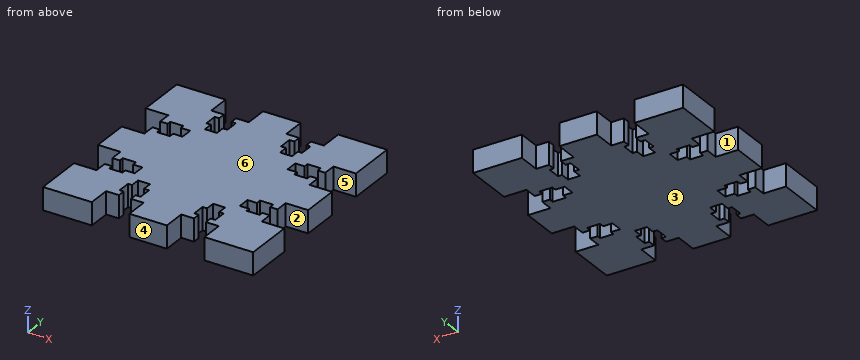
from build123d import *

# Parameters (mm, degrees)
SKETCH1_W           = 56
SKETCH1_H           = 56
BOSS_EXTRUDE1_DEPTH = 6
SKETCH2_W           = 10
SKETCH2_H           = 6
SKETCH2_W_2         = 6
SKETCH2_H_2         = 10
CUT_EXTRUDE1_DEPTH  = 54.425204723
SKETCH4_W           = 3.2
SKETCH4_H           = 6
CUT_EXTRUDE2_DEPTH  = 8
SKETCH10_W          = 6
SKETCH10_H          = 3.2
CUT_EXTRUDE7_DEPTH  = 8
SKETCH11_W          = 3.2
SKETCH11_H          = 6
CUT_EXTRUDE8_DEPTH  = 8
SKETCH12_W          = 6
SKETCH12_H          = 3.2
CUT_EXTRUDE9_DEPTH  = 8
SKETCH13_W          = 3.5
SKETCH13_H          = 5.6
SKETCH13_W_2        = 5.6
SKETCH13_H_2        = 3.5
CUT_EXTRUDE10_DEPTH = 54.425204723


with BuildPart() as part:
    # Sketch1 → Boss-Extrude1 (new body)
    with BuildSketch(Plane.XY):
        with Locations((6.733082315, -12.148044693)):
            Rectangle(SKETCH1_W, SKETCH1_H)
    extrude(amount=BOSS_EXTRUDE1_DEPTH)

    # Sketch2 → Cut-Extrude1 (cut, through all)
    with BuildSketch(Plane.XY.offset(6)):
        with Locations((-3.266917685, 12.851955307)):
            Rectangle(SKETCH2_W, SKETCH2_H)
        with Locations((16.733082315, 12.851955307)):
            Rectangle(SKETCH2_W, SKETCH2_H)
        with Locations((31.733082315, -2.148044693)):
            Rectangle(SKETCH2_W_2, SKETCH2_H_2)
        with Locations((31.733082315, -22.148044693)):
            Rectangle(SKETCH2_W_2, SKETCH2_H_2)
        with Locations((16.733082315, -37.148044693)):
            Rectangle(SKETCH2_W, SKETCH2_H)
        with Locations((-3.266917685, -37.148044693)):
            Rectangle(SKETCH2_W, SKETCH2_H)
        with Locations((-18.266917685, -22.148044693)):
            Rectangle(SKETCH2_W_2, SKETCH2_H_2)
        with Locations((-18.266917685, -2.148044693)):
            Rectangle(SKETCH2_W_2, SKETCH2_H_2)
    extrude(amount=-CUT_EXTRUDE1_DEPTH, mode=Mode.SUBTRACT)

    # Sketch4 → Cut-Extrude2 (cut)
    with BuildSketch(Plane(origin=(0, 9.851955307, 0), x_dir=(1, 0, 0), z_dir=(0, 1, 0))):
        with Locations((16.733082315, -3)):
            Rectangle(SKETCH4_W, SKETCH4_H)
        with Locations((-3.266917685, -3)):
            Rectangle(SKETCH4_W, SKETCH4_H)
    extrude(amount=-CUT_EXTRUDE2_DEPTH, mode=Mode.SUBTRACT)

    # Sketch10 → Cut-Extrude7 (cut)
    with BuildSketch(Plane(origin=(28.733082315, 0, 0), x_dir=(0, 0, -1), z_dir=(1, 0, 0))):
        with Locations((-3, -2.148044693)):
            Rectangle(SKETCH10_W, SKETCH10_H)
        with Locations((-3, -22.148044693)):
            Rectangle(SKETCH10_W, SKETCH10_H)
    extrude(amount=-CUT_EXTRUDE7_DEPTH, mode=Mode.SUBTRACT)

    # Sketch11 → Cut-Extrude8 (cut)
    with BuildSketch(Plane.XZ.offset(34.148044693)):
        with Locations((16.733082315, 3)):
            Rectangle(SKETCH11_W, SKETCH11_H)
        with Locations((-3.266917685, 3)):
            Rectangle(SKETCH11_W, SKETCH11_H)
    extrude(amount=-CUT_EXTRUDE8_DEPTH, mode=Mode.SUBTRACT)

    # Sketch12 → Cut-Extrude9 (cut)
    with BuildSketch(Plane.ZY.offset(15.266917685)):
        with Locations((3, -2.148044693)):
            Rectangle(SKETCH12_W, SKETCH12_H)
        with Locations((3, -22.148044693)):
            Rectangle(SKETCH12_W, SKETCH12_H)
    extrude(amount=-CUT_EXTRUDE9_DEPTH, mode=Mode.SUBTRACT)

    # Sketch13 → Cut-Extrude10 (cut, through all)
    with BuildSketch(Plane(origin=(0, 0, 0), x_dir=(-1, 0, 0), z_dir=(0, 0, -1))):
        with Locations((-24.983082315, -22.025968928)):
            Rectangle(SKETCH13_W, SKETCH13_H)
        with Locations((-16.61100655, 6.101955307)):
            Rectangle(SKETCH13_W_2, SKETCH13_H_2)
        with Locations((-24.983082315, -2.148044693)):
            Rectangle(SKETCH13_W, SKETCH13_H)
        with Locations((3.266917685, 6.101955307)):
            Rectangle(SKETCH13_W_2, SKETCH13_H_2)
        with Locations((11.516917685, -2.270120458)):
            Rectangle(SKETCH13_W, SKETCH13_H)
        with Locations((11.516917685, -22.148044693)):
            Rectangle(SKETCH13_W, SKETCH13_H)
        with Locations((3.14484192, -30.398044693)):
            Rectangle(SKETCH13_W_2, SKETCH13_H_2)
        with Locations((-16.733082315, -30.398044693)):
            Rectangle(SKETCH13_W_2, SKETCH13_H_2)
    extrude(amount=-CUT_EXTRUDE10_DEPTH, mode=Mode.SUBTRACT)


solid = part.part
The model under review builds one solid part; all positions refer to its coordinate system, in mm. Face numbers are marked on the shaded views. A direction names the side the tool comes from. Round coordinates to 2 decimals unless told otherwise and drop trailing zeros. Write each loop counter-clockwise with the first axis right and the second up, starting at its lowest first coordinate (ties: lowest second). Pieces come first, ordered by that corner, then holes. Notation, with made-up numbers: M -35,50 L -11,50 A11 cw -11,56 Z; hole C -38,88 d1. An arc over 180 degrees is marked long. Use a Markdown table: item, result. Add a question column.
Q1. We need section C-C, the plane y = -1.5. State the section outline as (x, z) points.
Q2. To check wall thickness, follow line 1 (X direction, y = -27, z = 5.2); line 2 (X direction, y = -34, z = 3.95); line 3 (Y direction, x = -12.5, z = 2.3). State the ranges of each line that lie inside material, in increasing order.
Q3. We need section B-B, the plane x = -10.5. State the section outline as (y, z) points.
Q4. The part is to be moulded in two halves that separate along Y. For the marked faces 4, 5 and 6, say which applies: pulls with the +Y half, pulls with the -Y half, needs draft (parallel to the pull), parting line crosses it, or undercut.
Q5. We need section A-A, the plane y = 12. State the section outline as (x, z) points.
Q6. Insertion check: pin 1 (3 mm diameter, centred on x = -1.5, z = 4, fed in from +Y); pin 2 (2.5 mm diameter, centred on y = 1, z = 3, fed in from -X); pin 3 (1.6 mm diameter, centred on x = -3.5, z = 2, fed in from -Y). Each pin has a flat end and moves straight along its axis. Give the tip position at first contact, or say it passes through.
Q7. Machinability: for the marked faces 1, 2 and 3, which of the approach directions +Z, -Z, +X, -X, +Y, -Y give a long, thin tool a straight path to every point of the face, cutting with its end or side? Answer none if there is none.
Findings below:
| question | item | result |
|---|---|---|
| 1 | outline | M -7.27,0 L 20.73,0 L 20.73,6 L -7.27,6 Z |
| 2 | line 1 | x = -15.27 to -4.87, -1.67 to 15.13, 18.33 to 28.73 |
| 2 | line 2 | x = -21.27 to -4.87, -1.67 to 15.13, 18.33 to 34.73 |
| 2 | line 3 | y = -40.15 to -24.95, -19.35 to -5.07, 0.53 to 15.85 |
| 3 | outline | M -40.15,0 L -24.95,0 L -24.95,6 L -40.15,6 Z; M -19.35,0 L -5.07,0 L -5.07,6 L -19.35,6 Z; M 0.53,0 L 15.85,0 L 15.85,6 L 0.53,6 Z |
| 4 | face 4 | pulls with the -Y half |
| 4 | face 5 | undercut |
| 4 | face 6 | needs draft |
| 5 | outline | M -21.27,0 L -8.27,0 L -8.27,6 L -21.27,6 Z; M 1.73,0 L 11.73,0 L 11.73,6 L 1.73,6 Z; M 21.73,0 L 34.73,0 L 34.73,6 L 21.73,6 Z |
| 6 | pin 1 | stops at y = 9.85 |
| 6 | pin 2 | stops at x = -15.27 |
| 6 | pin 3 | stops at y = -26.15 |
| 7 | face 1 | +Z, -Z, -X |
| 7 | face 2 | +Z, -Z, +X |
| 7 | face 3 | -Z, +X, -X, +Y, -Y |
